from build123d import *

# Parameters (mm, degrees)
F0_R     = 4
F1_DEPTH = 2.5


with BuildPart() as f1:
    # F0 (on Front) → F1 (new body, symmetric)
    with BuildSketch(Plane.XZ):
        with BuildLine():
            Line((24.9936, 9.8298), (0, 9.8298))
            Line((0, 9.8298), (-24.9936, 9.8298))
            ThreePointArc((-24.9936, 9.8298), (-34.8234, 0), (-24.9936, -9.8298))
            Line((-24.9936, -9.8298), (0, -9.8298))
            Line((0, -9.8298), (24.9936, -9.8298))
            ThreePointArc((24.9936, -9.8298), (34.8234, 0), (24.9936, 9.8298))
        make_face()
        with Locations((-24.9936, 0)):
            Circle(F0_R, mode=Mode.SUBTRACT)
        with BuildLine():
            ThreePointArc((28.9936, 0), (24.9936, -4), (20.9936, 0))
            ThreePointArc((20.9936, 0), (24.9936, 4), (28.9936, 0))
        make_face(mode=Mode.SUBTRACT)
    extrude(amount=F1_DEPTH, both=True)


solid = f1.part
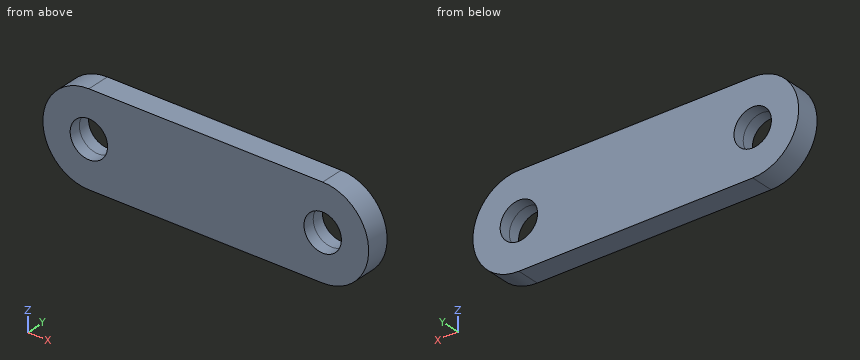
Check sheet for the modelled part. Datum: model origin and axes. Units: mm. Round coordinates to 2 decimals unless told otherwise and drop trailing zeros. Order: outer loops, then holes, each group sorted by start corner. A loop starts at its lowest first (then second) coordinate and runs counter-clockwise, first axis right, second up. Notation, with made-up numbers: M -18.75,-7.5 L 1.25,-7.5 A22 ccw 1.25,6.5 Z; hole C -39,-5.75 d10. An arc over 180 degrees is marked long. One line per item, written item: value. Start each with the question number.
1. Gauge pin test, flat ends, axial feed: P1, Ø3, axis at y = 1.5, z = 2.5, coming from the +X side; P2, Ø7, axis at x = 24.99, z = 0, coming from the +Y side (3 decimals). Record the tip position at first contact, or that the pin passes through.
2. Scan lines: line 1 along X through (y, z) = (-0.85, -0.75); line 2 along X through (y, z) = (-0.45, 3); line 3 along Z through (x, y) = (23.5, -2.15). Record each from-to range of solid material in increasing order.
3. Section check B-B on y = 1.8. Enter the section's corners in (x, z).
4. Section check D-D on x = -30. Enter the section's corners in (y, z).
5. Section check C-C on z = 5.75. Enter the section's corners in (x, y), and give its area (3 significant figures).
6. Section check A-A on z = 0. Enter the section's corners in (x, y).
Results found:
1. P1: x = 34.77
1. P2: through
2. line 1: -34.79 to -28.92, -21.06 to 21.06, 28.92 to 34.79
2. line 2: -34.35 to -27.64, -22.35 to 22.35, 27.64 to 34.35
2. line 3: -9.83 to -3.71, 3.71 to 9.83
3. outline: M -24.99,-9.83 L 24.99,-9.83 A9.83 ccw 24.99,9.83 L -24.99,9.83 A9.83 ccw Z; hole C -24.99,0 d8; hole C 24.99,0 d8
4. outline: M -2.5,-8.46 L 2.5,-8.46 L 2.5,8.46 L -2.5,8.46 Z
5. outline: M -32.97,-2.5 L 32.97,-2.5 L 32.97,2.5 L -32.97,2.5 Z
5. area: 330 mm^2
6. outline: M -34.82,-2.5 L -28.99,-2.5 L -28.99,2.5 L -34.82,2.5 Z; M -20.99,-2.5 L 20.99,-2.5 L 20.99,2.5 L -20.99,2.5 Z; M 28.99,-2.5 L 34.82,-2.5 L 34.82,2.5 L 28.99,2.5 Z
